Part model, mm, in its own coordinate system. Face numbers are marked on the shaded views. Coordinates: 2 decimals unless noted, no trailing zeros. Loops run counter-clockwise (first coordinate to the right, second up) from the corner with the lowest first, then second, coordinate; pieces in that order, holes last. Notation, with made-up numbers: M 75.25,38 L 129.25,38 A8 cw 129.25,49 Z; hole C -29,-24.75 d10. An arc over 180 degrees is marked long. Answer as a JSON object with one key per item and string values. Group by question number.
1. Drop flat-ended pins along their axis: pin 1 Ø2 at (y, z) = (-4.5, -8) entering from -X; pin 2 Ø4 at (x, z) = (-24, -6) entering from -Y (3 decimals); pin 3 Ø6 at (x, z) = (25.4, 0) entering from -Y. Give the stop position or say it passes through.
2. Saw through at B-B on z = -9. Write the cut outline in (x, y) (3 decimals), then the cut area to 3 significant figures.
3. Saw through at A-A on x = 0. Write the cut outline in (y, z).
4. Drill centre lines: L1, parallel to X at y = -0.25, z = -1; L2, parallel to Z at x = -0.5, y = -5.25; L3, parallel to X at y = -3, z = 6. Where is each one in solid material? Low to high.
5. Saw through at C-C on x = -25.4. Write the cut outline in (y, z) (3 decimals), then the cut area to 3 significant figures.
6. Mould opens along X. For the marked faces 1 and 2 say: released by +X, released by -X, zero draft, split by the parting line, or undercut.
7. Saw through at D-D on x = -15.5. Write the cut outline in (y, z) (3 decimals).
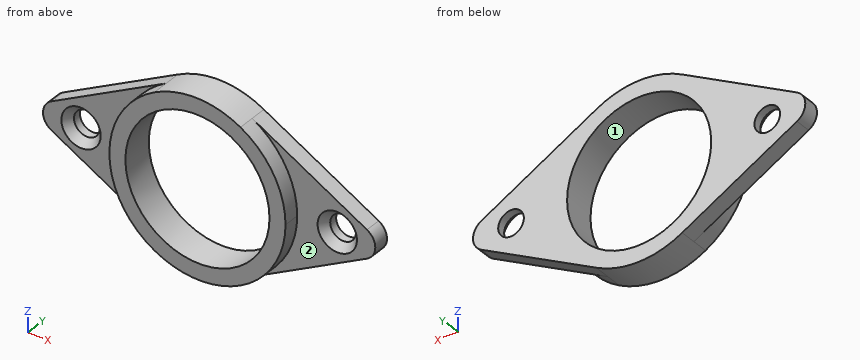
from build123d import *

# Parameters (mm, degrees)
F0_R           = 14.2875
F1_DEPTH       = 3.175
F2_DEPTH       = 6.35
F4_D           = 5.08
F4_CSINK_D     = 7.7978
F4_CSINK_ANGLE = 82


with BuildPart() as f1:
    # F0 (on Front) → F1 (new body)
    with BuildSketch(Plane.XZ):
        with BuildLine():
            ThreePointArc((8.525333, -15.24), (15.063408, -8.833608), (17.4625, 0))
            ThreePointArc((17.4625, 0), (15.063408, 8.833608), (8.525333, 15.24))
            ThreePointArc((8.525333, 15.24), (0, 17.4625), (-8.525333, 15.24))
            ThreePointArc((-8.525333, 15.24), (-17.4625, 0), (-8.525333, -15.24))
            ThreePointArc((-8.525333, -15.24), (0, -17.4625), (8.525333, -15.24))
        make_face()
        Circle(F0_R, mode=Mode.SUBTRACT)
        with BuildLine():
            ThreePointArc((8.525333, 15.24), (15.063408, 8.833608), (17.4625, 0))
            ThreePointArc((17.4625, 0), (15.063408, -8.833608), (8.525333, -15.24))
            Line((8.525333, -15.24), (31.288024, -2.785327))
            ThreePointArc((31.288024, -2.785327), (32.939024, 0), (31.288024, 2.785327))
            Line((31.288024, 2.785327), (8.525333, 15.24))
        make_face()
        with BuildLine():
            ThreePointArc((-8.525333, -15.24), (-17.4625, 0), (-8.525333, 15.24))
            Line((-8.525333, 15.24), (-31.288024, 2.785327))
            ThreePointArc((-31.288024, 2.785327), (-32.939024, 0), (-31.288024, -2.785327))
            Line((-31.288024, -2.785327), (-8.525333, -15.24))
        make_face()
    extrude(amount=F1_DEPTH)

    # F0 (on Front) → F2 (join)
    with BuildSketch(Plane.XZ):
        with BuildLine():
            ThreePointArc((8.525333, -15.24), (15.063408, -8.833608), (17.4625, 0))
            ThreePointArc((17.4625, 0), (15.063408, 8.833608), (8.525333, 15.24))
            ThreePointArc((8.525333, 15.24), (0, 17.4625), (-8.525333, 15.24))
            ThreePointArc((-8.525333, 15.24), (-17.4625, 0), (-8.525333, -15.24))
            ThreePointArc((-8.525333, -15.24), (0, -17.4625), (8.525333, -15.24))
        make_face()
        Circle(F0_R, mode=Mode.SUBTRACT)
    extrude(amount=F2_DEPTH)

    # F4 (through all)
    with Locations(Plane.XZ.offset(3.175)):
        with Locations((-25.4, 0), (25.4, 0)):
            CounterSinkHole(F4_D / 2, F4_CSINK_D / 2, counter_sink_angle=F4_CSINK_ANGLE)


solid = f1.part
Outcome:
{
 "1": {"pin 1": "stops at x = -16", "pin 2": "stops at y = -3.175", "pin 3": "stops at y = -2.14"},
 "2": {"outline": "M -19.93,-3.175 L -14.965,-3.175 L -14.965,-6.35 L -11.097,-6.35 L -11.097,0 L -19.93,0 Z; M 11.097,-6.35 L 14.965,-6.35 L 14.965,-3.175 L 19.93,-3.175 L 19.93,0 L 11.097,0 Z", "area": "80.7 mm²"},
 "3": {"outline": "M -6.35,-17.46 L 0,-17.46 L 0,-14.29 L -6.35,-14.29 Z; M -6.35,14.29 L 0,14.29 L 0,17.46 L -6.35,17.46 Z"},
 "4": {"L1": "x = -32.78 to -27.73, -23.07 to -14.25, 14.25 to 23.07, 27.73 to 32.78", "L2": "z = -17.46 to -14.28, 14.28 to 17.46", "L3": "x = -25.41 to -12.97, 12.97 to 25.41"},
 "5": {"outline": "M -3.175,-6.007 L 0,-6.007 L 0,-2.54 L -1.612,-2.54 L -3.175,-3.899 Z; M -3.175,3.899 L -1.612,2.54 L 0,2.54 L 0,6.007 L -3.175,6.007 Z", "area": "19.9 mm²"},
 "6": {"face 1": "undercut", "face 2": "zero draft"},
 "7": {"outline": "M -6.35,-8.043 L -3.175,-8.043 L -3.175,-11.424 L 0,-11.424 L 0,11.424 L -3.175,11.424 L -3.175,8.043 L -6.35,8.043 Z"}
}
